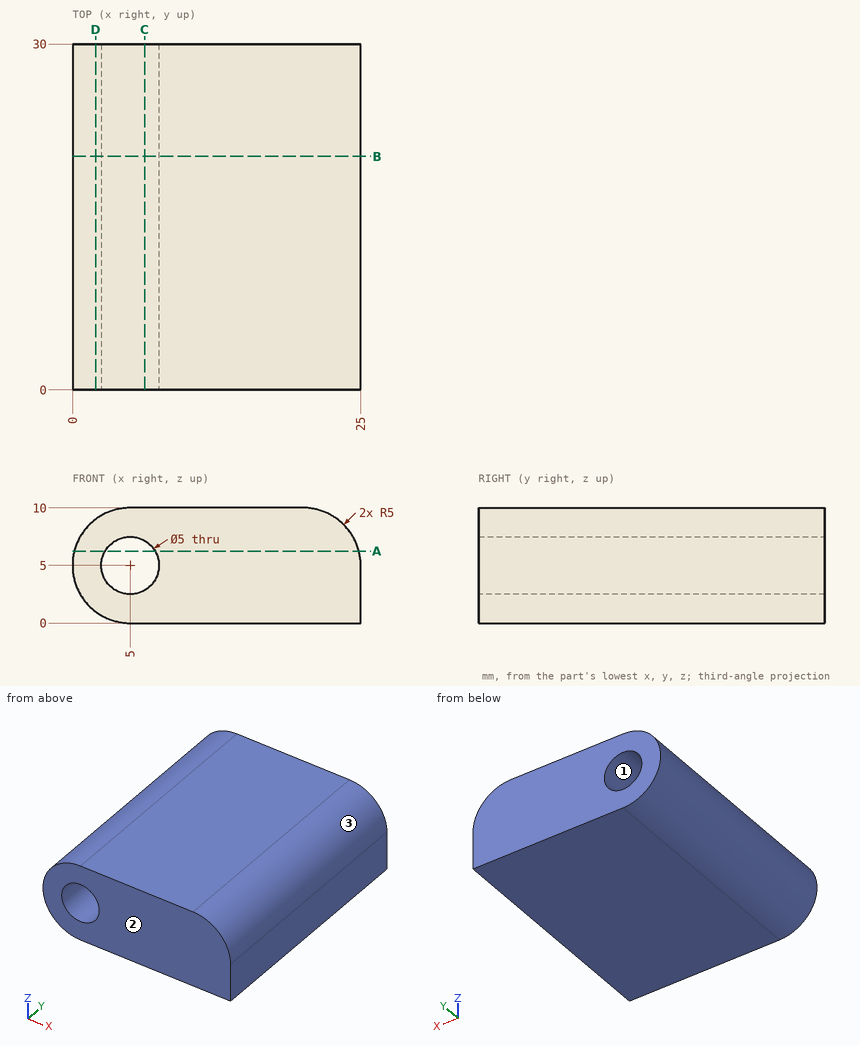
Study the drawing (mm; zero at the part's minimum x, y, z) and answer. Coordinates: 2 decimals unless noted, no trailing zeros. Write each loop counter-clockwise with the first axis right and the second up, starting at its lowest first coordinate (ties: lowest second). Pieces come first, ordered by that corner, then holes.
Q1. Determine the mould class of the marked faces 1, 2 and 3 for opening direction Z: released by +Z, released by -Z, zero draft, split by the parting line, or undercut.
Q2. A cutting plane is placed at D-D, the plane x = 2. Give the vertices of the cut face in (y, z), then the cut area to 3 significant figures.
Q3. A cutting plane is placed at B-B, the plane y = 20.25. Give the vertices of the cut face in (x, z).
Q4. A cutting plane is placed at C-C, the plane x = 6.25. Give the vertices of the cut face in (y, z), then the cut area to 3 significant figures.
Q5. A cutting plane is placed at A-A, the plane z = 6.25. Give the vertices of the cut face in (x, y), then the cut area to 3 significant figures.
Q6. Each of these flat-tipped pins is pushed along its axis until it touches: pin 1 Ø8 at (x, y) = (6, 27) entering from -Z; pin 2 Ø4 at (y, z) = (17.5, 8) entering from -X; pin 3 Ø3 at (x, z) = (5, 5) entering from +Y. Where does it stop, or does it pass through?
Q7. Find the intervals of material crossed by line 1 (X direction, y = 8.25, z = 3.75); line 2 (X direction, y = 22.25, z = 4.75); line 3 (X direction, y = 1.5, z = 9.25), in increasing order.
Findings below:
1. face 1: undercut
1. face 2: zero draft
1. face 3: released by +Z
2. outline: (0, 1) - (30, 1) - (30, 9) - (0, 9) - close
2. area: 240 mm2
3. outline: (5, 0) - (25, 0) - (25, 5) arc R5 ccw to (20, 10) - (5, 10) arc R5 ccw to start; hole circle Ø5 at (5, 5)
4. outline: (0, 0) - (30, 0) - (30, 2.83) - (0, 2.83) - close; (0, 7.17) - (30, 7.17) - (30, 10) - (0, 10) - close
4. area: 170 mm2
5. outline: (0.16, 0) - (2.83, 0) - (2.83, 30) - (0.16, 30) - close; (7.17, 0) - (24.84, 0) - (24.84, 30) - (7.17, 30) - close
5. area: 611 mm2
6. pin 1: stops at z = 0
6. pin 2: stops at x = 0.1
6. pin 3: passes through
7. line 1: x = 0.16 to 2.83, 7.17 to 25
7. line 2: x = 0.01 to 2.51, 7.49 to 25
7. line 3: x = 2.37 to 22.63
